Autodesk Inventor part; units mm, degrees
ref_plane "YZ Plane" through (0, 0, 0) normal (1, 0, 0) x (0, 1, 0)
ref_plane "XZ Plane" through (0, 0, 0) normal (0, 1, 0) x (-1, 0, 0)
ref_plane "XY Plane" through (0, 0, 0) normal (0, 0, 1) x (1, 0, 0)
sketch "Sketch1" plane through (0, 0, 0) normal (0, 1, 0) x (-1, 0, 0)
  line L0 (0, 0) -> (50, 0)
  line L1 (50, 0) -> (50, -100)
  line L2 (50, -100) -> (0, -100)
  line L3 (0, -100) -> (0, 0)
  line L4 (25, 0) -> (25, -100)
  line L5 (7.5, -54) -> (7.5, -10)
  line L6 (7.5, -10) -> (42.5, -10)
  line L7 (42.5, -10) -> (42.5, -54)
  line L8 (42.5, -54) -> (7.5, -54)
  line L9 (7.5, -54) -> (42.5, -10) construction
  line L10 (7.5, -10) -> (42.5, -54) construction
  line L11 (7.5, -54) -> (51.5, -54) construction
  line L12 (14.75, -64.45) -> (14.75, -89.55)
  line L13 (14.75, -89.55) -> (35.25, -89.55)
  line L14 (35.25, -89.55) -> (35.25, -64.45)
  line L15 (35.25, -64.45) -> (14.75, -64.45)
  line L16 (14.75, -64.45) -> (35.25, -89.55) construction
  line L17 (14.75, -89.55) -> (35.25, -64.45) construction
  line L18 (14.75, -64.45) -> (39.85, -64.45) construction
  line L19 (25, -10) -> (25, -15)
  line L20 (25, -10) -> (30, -10) construction
  line L21 (20, -20) -> (30, -20)
  line L22 (30, -20) -> (30, -10)
  line L23 (30, -10) -> (20, -10)
  line L24 (20, -10) -> (20, -20)
  line L25 (20, -20) -> (30, -10) construction
  line L26 (30, -20) -> (20, -10) construction
  line L27 (20, -20) -> (30, -20) construction
  line L28 (30, -15) -> (20, -15)
  line L29 (20, -10) -> (30, -10)
  line L30 (30, -10) -> (30, -5)
  line L31 (30, -5) -> (20, -5)
  line L32 (20, -5) -> (20, -10)
  line L33 (25, -54) -> (25, -64.45)
  line L34 (30, -54) -> (30, -64.45)
  line L35 (30, -64.45) -> (20, -64.45)
  line L36 (20, -64.45) -> (20, -54)
  line L37 (20, -54) -> (30, -54)
  line L38 (30, -54) -> (20, -64.45) construction
  line L39 (30, -64.45) -> (20, -54) construction
  circle A0 centre (25, -31.5) radius 22.5
  point P0 (25, -32)
  point P1 (25, -77)
  point P2 (25, -77)
  point P3 (25, -59.225)
  dimension "d36" = 45
  dimension "d0" = 50
  dimension "d1" = 100
  dimension "d2" = 44
  dimension "d3" = 90
  dimension "d4" = 35
  dimension "d5" = 10
  dimension "d6" = 25.1
  dimension "d7" = 90
  dimension "d8" = 20.5
  dimension "d9" = 5
  dimension "d10" = 90
  dimension "d11" = 0
  dimension "d23" = 10
  dimension "d24" = 5
  dimension "d25" = 10
extrude "Extrusion1" add sketch "Sketch1" along normal blind 10
ref_plane "Work Plane1" through (-14.75, 0, -89.55) normal (0, 0, -1) x (-1, 0, 0)
ref_plane "Work Plane2" through (-14.75, 0, -64.45) normal (0, 0, -1) x (-1, 0, 0)
ref_plane "Work Plane3" through (-7.5, 0, -54) normal (0, 0, -1) x (-1, 0, 0)
ref_plane "Work Plane4" through (-7.5, 0, -10) normal (0, 0, -1) x (-1, 0, 0)
sketch "Sketch2" plane through (-14.75, 0, -89.55) normal (0, 0, -1) x (-1, 0, 0)
  line L0 (-14.75, 0) -> (35.25, 0)
  line L1 (35.25, 0) -> (35.25, 10)
  line L2 (-14.75, 10) -> (35.25, 10)
  line L3 (-14.75, 0) -> (-14.75, 10)
  line L4 (-14.75, 0) -> (35.25, 0)
  line L5 (35.25, 0) -> (35.25, -50)
  line L6 (35.25, -50) -> (-14.75, -50)
  line L7 (-14.75, -50) -> (-14.75, 0)
  line L8 (0, 0) -> (20.5, 0)
  circle A0 centre (10.25, -25) radius 10.25
  dimension "d14" = 50
  dimension "d15" = 50
  dimension "d16" = 20.5
sketch "Sketch3" plane through (-7.5, 0, -54) normal (0, 0, -1) x (-1, 0, 0)
  line L0 (42.5, 0) -> (-7.5, 0)
  line L1 (-7.5, 0) -> (-7.5, 10)
  line L2 (42.5, 10) -> (-7.5, 10)
  line L3 (42.5, 0) -> (42.5, 10)
  line L4 (-7.5, 0) -> (42.5, 0)
  line L5 (42.5, 0) -> (42.5, -50)
  line L6 (42.5, -50) -> (-7.5, -50)
  line L7 (-7.5, -50) -> (-7.5, 0)
  line L8 (0, 0) -> (35, 0)
  circle A0 centre (17.5, -25) radius 17.5
  dimension "d17" = 50
  dimension "d18" = 50
  dimension "d19" = 35
sketch "Sketch4" plane through (-14.75, 0, -64.45) normal (0, 0, -1) x (-1, 0, 0)
  line L0 (35.25, 0) -> (-14.75, 0)
  line L1 (-14.75, 0) -> (-14.75, 10)
  line L2 (35.25, 10) -> (-14.75, 10)
  line L3 (35.25, 0) -> (35.25, 10)
  line L4 (-14.75, 0) -> (35.25, 0)
  line L5 (35.25, 0) -> (35.25, -50)
  line L6 (35.25, -50) -> (-14.75, -50)
  line L7 (-14.75, -50) -> (-14.75, 0)
  circle A0 centre (10.25, -25) radius 5
  dimension "d20" = 50
  dimension "d21" = 50
  dimension "d22" = 10
ref_plane "Work Plane5" through (-25, -25, -89.55) normal (0, -1, 0) x (1, 0, 0)
extrude "Extrusion2" add sketch "Sketch1" against normal up to surface (25 mm away) contours L31 L30 A0 L4 | L4 A0 L32 L31 | A0 L30 L6 L4 | L4 L6 L32 A0 | L13 L12 L15 L4 | L4 L15 L14 L13 | L6 L22 L28 L4 | L4 L28 L24 L6 | L15 L36 L8 L4 | L4 L8 L34 L15 | L28 L22 L21 L4 | L4 L21 L24 L28 | L24 L21 L4 A0 L5 L6 | L6 A0 L7 L4 L21 L22 | L6 L7 A0 | A0 L5 L6 | A0 L7 L8 | L8 L5 A0
extrude "Extrusion3" cut sketch "Sketch2" against normal up to surface (25.1 mm away) contours A0
ref_plane "Work Plane6" through (-30, -25, -5) normal (0, 0, 1) x (1, 0, 0)
extrude "Extrusion4" cut sketch "Sketch4" against normal up to surface (59.45 mm away) contours A0
extrude "Extrusion5" cut sketch "Sketch3" against normal up to surface (49 mm away) contours A0
extrude "Extrusion6" cut sketch "Sketch1" along normal up to surface (10 mm away) contours A0 L30 L6 L4 | L4 L6 L32 A0 | L6 L22 L28 L4 | L4 L28 L24 L6 | A0 L6 L30 | L32 L6 A0 | L28 L22 L21 L4 | L4 L21 L24 L28 | L24 L21 L4 A0 L5 L6 | L6 A0 L7 L4 L21 L22 | A0 L7 | L5 A0
properties part number "dcmotor_housing_lid"
Model file for the job. Use its own axes, mm. A direction names the side the tool comes from. Give positions to 0.01 mm unless a question says otherwise; leave off trailing zeros. Write each loop counter-clockwise with the first axis right and the second up, starting at its lowest first coordinate (ties: lowest second). Pieces come first, ordered by that corner, then holes. Notation, with made-up numbers: (-19.5, 65) - (27.5, 65) arc R17 ccw to (27.5, 93) - close; hole circle Ø8 at (81.5, 28). An arc over 180 degrees is marked (long way). One line per question, with ' | ' between items. Start each with the question number.
(1) Slice it at A-A on z = -31.5. Write the cut outline in (x, y), plus the area to 3 significant figures.
(2) Slice it at C-C on x = -25. Write the cut outline in (y, z).
(3) 3-axis set-ups, long thin cutter, end or side, ignore diameter. For faces 1 (the face through (-25.385, -7.504, -29.843)), 2 (the face through (-25, -19, -64.45)), 3 (the face through (-12, -7, -10)), 4 (the face through (-12, -7, -54)): which of +Z, -Z, +X, -X, +Y, -Y reach the whole face in a straight line?
(4) Slice it at D-D on z = -65.5. Write the cut outline in (x, y).
(5) Pin check, flat tips, straight feed: P1, Ø4, axis at y = -4, z = -6.5, coming from the +X side; P2, Ø5, axis at x = -25.5, y = -13, coming from the +Z side; P3, Ø5, axis at x = -9.5, z = -77, coming from the -Y side. Stop position of each tip, or through.
(6) Slice it at B-B on y = -3. Write the cut outline in (x, z).
(7) Wall check: line 1 along X through (y, z) = (3, -31.5); line 2 along Y through (x, z) = (-36.5, -65); line 3 along Z through (x, y) = (-25, 8). Give the ranges that are in metal, low to high. Write a range as from..to.
(8) Two-plate mould, pull along X, no slides. Class faces 5 (the face through (0, 5, -51)), 6 (the face through (-25, 0, -31)), 7 (the face through (-35.25, -12, -77)): +X half, -X half, draft (parallel to the pull), parting line (faces both ways), or undercut.
Results below:
1) outline: (-50, 0) - (-47.5, 0) - (-47.5, 10) - (-50, 10) - close; (-42.5, -25) arc R17.5 cw to (-7.5, -25) - (-7.5, 0) - (-42.5, 0) - close; (-2.5, 0) - (0, 0) - (0, 10) - (-2.5, 10) - close | area: 444 mm^2
2) outline: (-20, -64.45) - (-14.75, -64.45) - (-14.75, -89.55) - (0, -89.55) - (0, -100) - (10, -100) - (10, -54) - (0, -54) - (0, -9) - (10, -9) - (10, 0) - (0, 0) - (0, -5) - (-7.5, -5) - (-7.5, -54) - (-20, -54) - close
3) face 1: +Z, -Y | face 2: -Z, -Y | face 3: +Z, +X, -Y | face 4: +X, -Y
4) outline: (-50, 0) - (-35.25, 0) - (-35.25, -25) arc R10.25 cw to (-14.75, -25) - (-14.75, 0) - (0, 0) - (0, 10) - (-50, 10) - close
5) P1: x = -20 | P2: z = -54 | P3: y = 0
6) outline: (-42.5, -54) - (-30, -54) - (-30, -64.45) - (-35.25, -64.45) - (-35.25, -89.55) - (-14.75, -89.55) - (-14.75, -64.45) - (-20, -64.45) - (-20, -54) - (-7.5, -54) - (-7.5, -10) - (-20, -10) - (-20, -5) - (-30, -5) - (-30, -10) - (-42.5, -10) - close
7) line 1: -50..-47.5, -2.5..0 | line 2: 0..10 | line 3: -100..-54, -9..0
8) face 5: +X half | face 6: undercut | face 7: -X half
